The figure shows three views and two pictorial views of one solid part (mm, origin at its lowest corner). Answer the questions. Round coordinates to 2 decimals unless told otherwise and drop trailing zeros. Write each loop counter-clockwise with the first axis right and the second up, starting at its lowest first coordinate (ties: lowest second). Pieces come first, ordered by that corner, then holes. Notation, with made-up numbers: (77, -11) -> (103, -11) arc R20 ccw to (103, 9) -> close; hole circle Ø5 at (-31, 50). An arc over 180 degrees is marked (long way). One line per item, written item: value.
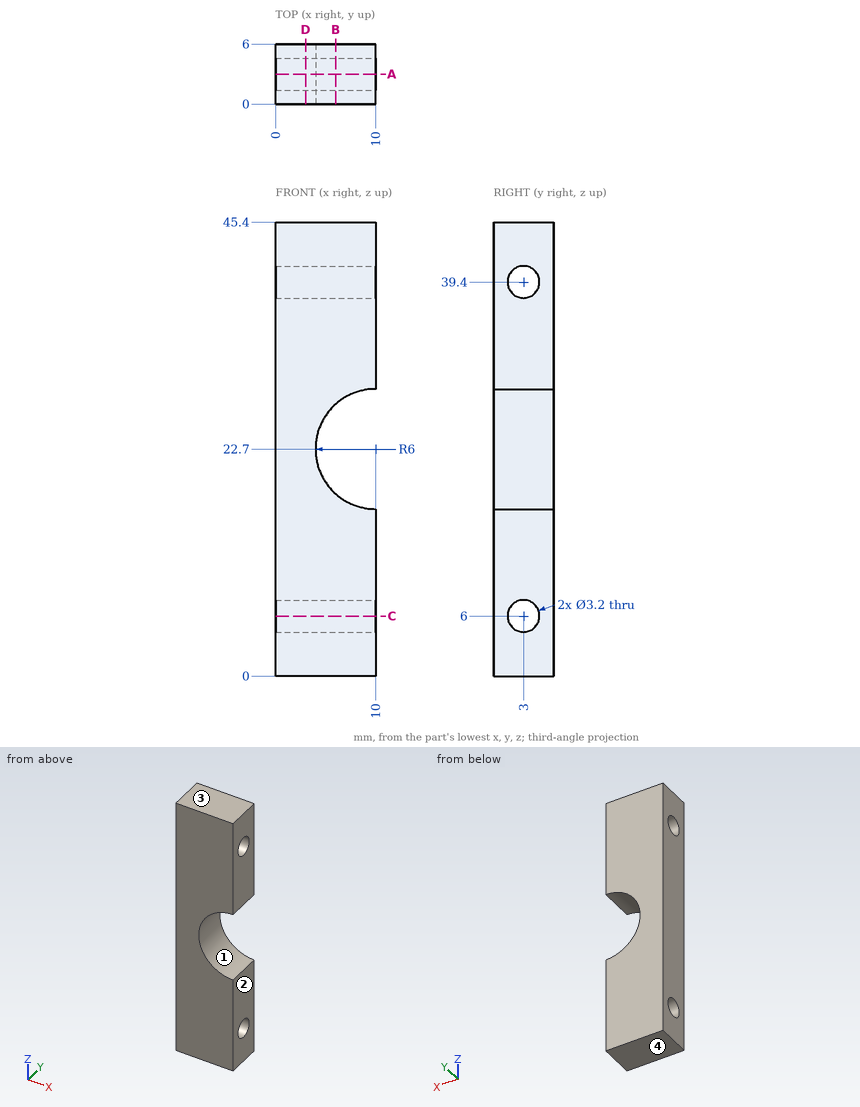
(1) Find section D-D on x = 3. Give the vertices of the cut face in (y, z), plus the area to 3 significant figures.
Reported:
outline: (0, 0) -> (6, 0) -> (6, 45.4) -> (0, 45.4) -> close; hole circle Ø3.2 at (3, 6); hole circle Ø3.2 at (3, 39.4)
area: 256 mm2
(2) A flat-ended cylindrical pin translates along its axis: pin 1 Ø2.5 at (y, z) = (3, 6) entering from +X. Find the tip coordinate at first contact, or state that the pin passes through.
Reported:
pin 1: passes through
(3) For a pull along Z with two mould halves and no side action, classify the marked faces 1, 2, 3 and 4 as pulls with the +Z half, pulls with the -Z half, needs draft (parallel to the pull), parting line crosses it, or undercut.
Reported:
face 1: undercut
face 2: needs draft
face 3: pulls with the +Z half
face 4: pulls with the -Z half
(4) Consider probe 1 along Z at (x, y) = (3.5, 2.5); probe 2 along Z at (x, y) = (3.5, 2.3); probe 3 along Y at (x, z) = (6.75, 39.4). Determine where each line is inside the solid, lowest interval first.
Reported:
probe 1: z = 0 to 4.48, 7.52 to 37.88, 40.92 to 45.4
probe 2: z = 0 to 4.56, 7.44 to 37.96, 40.84 to 45.4
probe 3: y = 0 to 1.4, 4.6 to 6
(5) Find section C-C on z = 6. Give the vertices of the cut face in (x, y).
Reported:
outline: (0, 0) -> (10, 0) -> (10, 1.4) -> (0, 1.4) -> close; (0, 4.6) -> (10, 4.6) -> (10, 6) -> (0, 6) -> close
(6) Find section A-A on y = 3. Give the vertices of the cut face in (x, z).
Reported:
outline: (0, 0) -> (10, 0) -> (10, 4.4) -> (0, 4.4) -> close; (0, 7.6) -> (10, 7.6) -> (10, 16.7) arc R6 cw to (10, 28.7) -> (10, 37.8) -> (0, 37.8) -> close; (0, 41) -> (10, 41) -> (10, 45.4) -> (0, 45.4) -> close
(7) Find section B-B on x = 6. Give the vertices of the cut face in (y, z).
Reported:
outline: (0, 0) -> (6, 0) -> (6, 18.23) -> (0, 18.23) -> close; (0, 27.17) -> (6, 27.17) -> (6, 45.4) -> (0, 45.4) -> close; hole circle Ø3.2 at (3, 6); hole circle Ø3.2 at (3, 39.4)
